Model file for the job. Use its own axes, mm. Face numbers are marked on the shaded views. Give positions to 0.01 mm unless a question says otherwise; leave off trailing zeros. Loops run counter-clockwise (first coordinate to the right, second up) from the corner with the lowest first, then second, coordinate; pieces in that order, holes last. Notation, with made-up numbers: (60, -14) - (109, -14) arc R18 cw to (109, 7) - close; hole circle Ø8 at (-4.75, 22.5). An arc over 180 degrees is marked (long way). Use a Markdown table: item, result.
Autodesk Inventor part; units mm, degrees
ref_plane "YZ Plane" through (0, 0, 0) normal (1, 0, 0) x (0, 1, 0)
ref_plane "XZ Plane" through (0, 0, 0) normal (0, 1, 0) x (-1, 0, 0)
sketch "Sketch1" plane through (0, 0, 0) normal (0, 0, 1) x (1, 0, 0)
  circle A0 centre (0, 0) radius 25
  dimension "d0" = 50
ref_plane "Work Plane1" through (0, 0, 250) normal (0, 0, 1) x (1, 0, 0)
sketch "Sketch2" plane through (0, 0, 250) normal (0, 0, 1) x (1, 0, 0)
  circle A0 centre (0, 0) radius 100
  line L0 (0, 0) -> (0, -169.491589)
  line L1 (-100, 0) -> (-100, -163.22364)
  dimension "d2" = 200
sketch "Sketch1 outline for Loft1" plane through (0, 0, 0) normal (0, 0, 1) x (1, 0, 0)
  circle A0 centre (0, 0) radius 25
sketch "Sketch2 outline for Loft1" plane through (0, 0, 250) normal (0, 0, 1) x (1, 0, 0)
  circle A0 centre (0, 0) radius 100
loft "Loft1" add profiles "Sketch1 outline for Loft1", "Sketch2 outline for Loft1"
ref_plane "Work Plane6" through (0, 0, 450) normal (0, 0, 1) x (1, 0, 0)
sketch "Sketch7" plane through (0, 0, 450) normal (0, 0, 1) x (1, 0, 0)
  circle A0 centre (0, 0) radius 75
  dimension "d15" = 150
sketch "Sketch7 outline for Loft2" plane through (0, 0, 450) normal (0, 0, 1) x (1, 0, 0)
  circle A0 centre (0, 0) radius 75
loft "Loft2" add profiles "Sketch7 outline for Loft2" section 1 edges at (-100, 0, 250)
ref_plane "Work Plane7" through (0, 0, 750) normal (0, 0, 1) x (1, 0, 0)
sketch "Sketch8" plane through (0, 0, 750) normal (0, 0, 1) x (1, 0, 0)
  line L0 (110.354309, -111.480379) -> (-110.354309, -111.480379)
  line L1 (-110.354309, -111.480379) -> (-110.354309, 111.480379)
  line L2 (-110.354309, 111.480379) -> (110.354309, 111.480379)
  line L3 (110.354309, 111.480379) -> (110.354309, -111.480379)
  line L4 (110.354309, -111.480379) -> (-110.354309, 111.480379) construction
  line L5 (-110.354309, -111.480379) -> (110.354309, 111.480379) construction
  point P0 (0, 0)
sketch "Sketch8 outline for Loft3" plane through (0, 0, 750) normal (0, 0, 1) x (1, 0, 0)
  line L0 (110.354309, -111.480379) -> (-110.354309, -111.480379)
  line L1 (-110.354309, -111.480379) -> (-110.354309, 111.480379)
  line L2 (-110.354309, 111.480379) -> (110.354309, 111.480379)
  line L3 (110.354309, 111.480379) -> (110.354309, -111.480379)
loft "Loft3" add profiles "Sketch8 outline for Loft3" section 1 edges at (-75, 0, 450)
properties part number "PartOne"
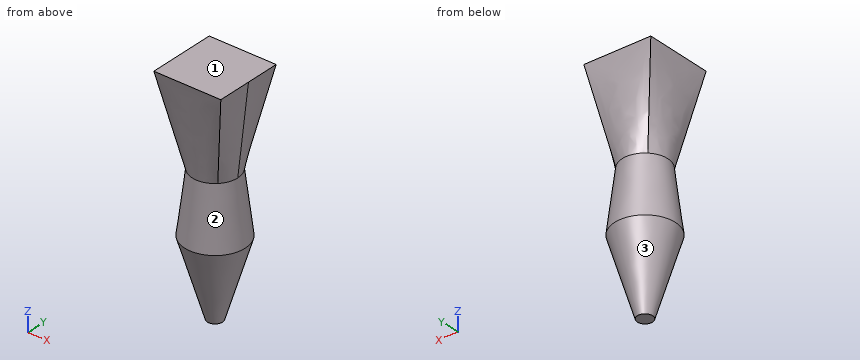
(1) Pin check, flat tips, straight feed: P1, Ø3, axis at x = 54.5, z = 152, coming from the +Y side; P2, Ø12, axis at x = 32.5, z = 407.5, coming from the -Y side; P3, Ø8, axis at y = 51.5, z = 361, coming from the +X side. Stop position of each tip, or through.
Computed:
| item | result |
|---|---|
| P1 | y = 46.77 |
| P2 | y = -75.96 |
| P3 | x = 71.91 |
(2) Slice it at A-A, the plane z = 143.5. Write the cut outline in (x, y).
Computed:
| item | result |
|---|---|
| outline | circle Ø136.1 at (0, 0) |
(3) Mould opens along Z. For the marked faces 1, 2 and 3 say: pulls with the +Z half, pulls with the -Z half, needs draft (parallel to the pull), parting line crosses it, or undercut.
Computed:
| item | result |
|---|---|
| face 1 | pulls with the +Z half |
| face 2 | undercut |
| face 3 | pulls with the -Z half |
(4) Drill centre lines: probe 1 along X at (y, z) = (-46.5, 448); probe 2 along X at (y, z) = (35, 352); probe 3 along Y at (x, z) = (36, 409). Where is each one in solid material? Low to high. Write a range as [from, to].
Computed:
| item | result |
|---|---|
| probe 1 | [-59.16, 59.16] |
| probe 2 | [-79.92, 79.92] |
| probe 3 | [-71.58, 71.58] |
